Study the drawing (mm; zero at the part's minimum x, y, z) and answer. Coordinates: 2 decimals unless noted, no trailing zeros. Loops run counter-clockwise (first coordinate to the right, second up) from the corner with the lowest first, then second, coordinate; pieces in that order, holes last. Notation, with made-up numbers: (57.5, -14) -> (79.5, -14) arc R11 ccw to (79.5, 3) -> close; hole circle Ø8 at (77.25, 70). An arc over 180 degrees is marked (long way). One line per question, with ' | ' between items. Start each with the question number.
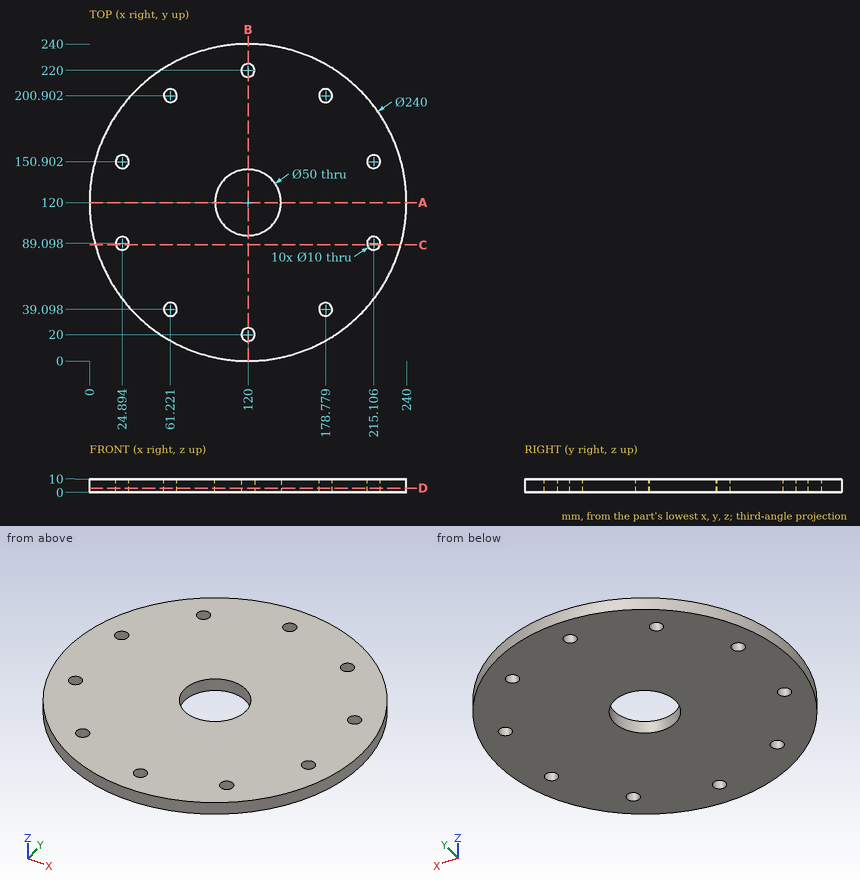
(1) Find the intervals of material crossed by probe 1 along Y at (x, z) = (62.5, 9) (1 decimal); probe 2 along X at (y, z) = (197.5, 6.25) (1 decimal); probe 3 along Y at (x, z) = (130, 1), in increasing order. Write a range as from..to.
(2) This flat-tipped pin is pushed along its axis until it touches: pin 1 Ø6 at (x, y) = (24.89, 150.9) entering from -Z. Where does it stop, or does it pass through?
(3) Section A-A on y = 120 is taken. Write down the section's boundary in (x, z), plus the area to 3 significant figures.
(4) Section D-D on z = 3 is taken. Give the number of separate pieces and of enclosed holes in the cut face, plus the area to 3 significant figures.
(5) Section C-C on y = 88 is taken. Write down the section's boundary in (x, z) (1 decimal), plus the area to 3 significant figures.
(6) Section B-B on x = 120 is taken. Write down the section's boundary in (y, z).
Working result:
1) probe 1: y = 14.7..34.3, 43.9..196.1, 205.7..225.3 | probe 2: x = 28.4..57.6, 64.9..175.1, 182.4..211.6 | probe 3: y = 0.42..97.09, 142.91..239.58
2) pin 1: passes through
3) outline: (0, 0) -> (95, 0) -> (95, 10) -> (0, 10) -> close; (145, 0) -> (240, 0) -> (240, 10) -> (145, 10) -> close | area: 1,900 mm2
4) separate pieces: 1 | enclosed holes: 11 | area: 42,500 mm2
5) outline: (4.3, 0) -> (20, 0) -> (20, 10) -> (4.3, 10) -> close; (29.8, 0) -> (210.2, 0) -> (210.2, 10) -> (29.8, 10) -> close; (220, 0) -> (235.7, 0) -> (235.7, 10) -> (220, 10) -> close | area: 2,120 mm2
6) outline: (0, 0) -> (15, 0) -> (15, 10) -> (0, 10) -> close; (25, 0) -> (95, 0) -> (95, 10) -> (25, 10) -> close; (145, 0) -> (215, 0) -> (215, 10) -> (145, 10) -> close; (225, 0) -> (240, 0) -> (240, 10) -> (225, 10) -> close
